Build history of the part. All positions in model axes, mm. Face numbers are marked on the shaded views. A direction names the side the tool comes from. Give positions to 0.01 mm unless a question says otherwise; leave off trailing zeros. Loops run counter-clockwise (first coordinate to the right, second up) from the corner with the lowest first, then second, coordinate; pieces in that order, holes last. Notation, with made-up numbers: (57.25, 63.25) -> (81.25, 63.25) arc R23 cw to (81.25, 99.25) -> close; hole circle Ø3 at (28.25, 58). An arc over 180 degrees is marked (long way). Answer as a JSON object with one key per item and string values. Group by question number.
Q1. Band-saw the part on D-D, the plane x = 9. Write the cut outline in (y, z).
Q2. Wall check: probe 1 along Y at (x, z) = (0, 2); probe 2 along X at (y, z) = (-6, 0.95); probe 3 along X at (y, z) = (-3.5, 0.4). Give the ranges that are in metal, low to high. Write a range as from..to.
Q3. Band-saw the part on A-A, the plane y = -6. Write the cut outline in (x, z), plus the area to 3 significant figures.
Q4. Band-saw the part on B-B, the plane x = 0. Write the cut outline in (y, z).
Q5. Band-saw the part on C-C, the plane z = 1.8. Write the cut outline in (x, y).
Q6. Drop a flat-ended pin along its axis: pin 1 (2.5 mm diameter, centred on x = 0, y = 11.5, fed in from -Z). Give the stop position or say it passes through.
Q7. Tool access for the marked faces 1, 2 and 3: list every direction of +Z, -Z, +X, -X, +Y, -Y with a clear straight run to the whole face (end or side of a thin tool).
Autodesk Inventor part; units mm, degrees
ref_plane "YZ Plane" through (0, 0, 0) normal (1, 0, 0) x (0, 1, 0)
ref_plane "XZ Plane" through (0, 0, 0) normal (0, 1, 0) x (-1, 0, 0)
ref_plane "XY Plane" through (0, 0, 0) normal (0, 0, 1) x (1, 0, 0)
sketch "Boceto1" plane through (0, 0, 0) normal (0, 0, 1) x (1, 0, 0)
  line L0 (-7.5, -16.5) -> (7.5, -16.5)
  line L1 (7.5, -16.5) -> (7.5, 16.5)
  line L2 (7.5, 16.5) -> (-7.5, 16.5)
  line L3 (-7.5, 16.5) -> (-7.5, -16.5)
  line L4 (-7.5, -16.5) -> (7.5, 16.5) construction
  line L5 (7.5, -16.5) -> (-7.5, 16.5) construction
  point P0 (0, 0)
  dimension "d7" = 33
  dimension "d8" = 15
extrude "Extrusión1" add sketch "Boceto1" along normal blind 3
sketch "Boceto2" plane through (0, 0, 0) normal (0, 0, -1) x (-1, 0, 0)
  line L0 (-20, -16.5) -> (20, -16.5)
  line L1 (20, -16.5) -> (20, -11.5)
  line L2 (20, -11.5) -> (-20, -11.5)
  line L3 (-20, -11.5) -> (-20, -16.5)
  point P0 (0, 0)
  point P1 (7.5, -16.5)
  dimension "d2" = 20
  dimension "d3" = 20
  dimension "d4" = 5
extrude "Extrusión2" add sketch "Boceto2" against normal blind 3
sketch "Boceto3" plane through (0, 0, 0) normal (0, 0, -1) x (-1, 0, 0)
  line L0 (-20, -16.5) -> (20, -16.5) construction
  point P0 (0, 0)
  point P1 (0, -6)
  point P2 (0, 11.5)
  dimension "d9" = 10.5
  dimension "d10" = 17.5
hole "Agujero1" at (0, -6, 0) at (0, 11.5, 0) direction (0, 0, 1) diameter 3 end through all
properties part number "Soporte_Motorreductor"
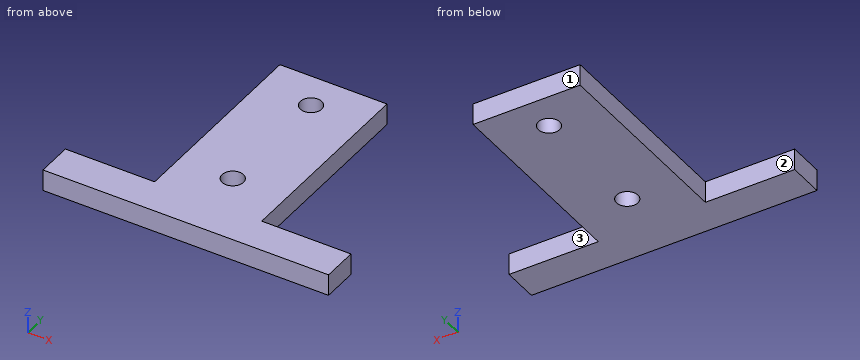
Worked answers:
{
 "1": {"outline": "(-16.5, 0) -> (-11.5, 0) -> (-11.5, 3) -> (-16.5, 3) -> close"},
 "2": {"probe 1": "-16.5..-7.5, -4.5..10, 13..16.5", "probe 2": "-7.5..-1.5, 1.5..7.5", "probe 3": "-7.5..7.5"},
 "3": {"outline": "(-7.5, 0) -> (-1.5, 0) -> (-1.5, 3) -> (-7.5, 3) -> close; (1.5, 0) -> (7.5, 0) -> (7.5, 3) -> (1.5, 3) -> close", "area": "36.0 mm2"},
 "4": {"outline": "(-16.5, 0) -> (-7.5, 0) -> (-7.5, 3) -> (-16.5, 3) -> close; (-4.5, 0) -> (10, 0) -> (10, 3) -> (-4.5, 3) -> close; (13, 0) -> (16.5, 0) -> (16.5, 3) -> (13, 3) -> close"},
 "5": {"outline": "(-20, -16.5) -> (20, -16.5) -> (20, -11.5) -> (7.5, -11.5) -> (7.5, 16.5) -> (-7.5, 16.5) -> (-7.5, -11.5) -> (-20, -11.5) -> close; hole circle Ø3 at (0, -6); hole circle Ø3 at (0, 11.5)"},
 "6": {"pin 1": "through"},
 "7": {"face 1": "+Z, -Z, +X, -X, +Y", "face 2": "+Z, -Z, -X, +Y", "face 3": "+Z, -Z, +X, +Y"}
}
